```python
from build123d import *
from build123d.topology import SkipClean

# Parameters (mm, degrees)
SKETCH1_R           = 11.1
SKETCH1_R_2         = 2.95
BOSS_EXTRUDE1_DEPTH = 6.4
CUT_EXTRUDE4_REACH  = 48.556
CHAMFER1_SIZE       = 1
CUT_EXTRUDE3_DEPTH  = 47.555734529
FILLET1_R           = 10
FILLET2_R           = 5
SKETCH7_R           = 11.1
SKETCH7_R_2         = 9.1
BOSS_EXTRUDE2_DEPTH = 0.4
SKETCH9_OUTSIDE_W   = 87.68
SKETCH9_OUTSIDE_H   = 55.695
SKETCH9_OUTSIDE_R   = 16
CUT_EXTRUDE5_DEPTH  = 0.4
CUT_EXTRUDE6_DEPTH  = 0.15
CHAMFER2_SIZE       = 0.4


with BuildPart() as part:
    # Sketch1 → Boss-Extrude1 (new body)
    with BuildSketch(Plane(origin=(0, 0, 0), x_dir=(1, 0, 0), z_dir=(0, 1, 0))):
        with BuildLine():
            Line((-9.621787606, -11.507441213), (-37.944538575, 12.174234774))
            ThreePointArc((-37.944538575, 12.174234774), (-39.566706632, 19.240834224), (-33.200130557, 22.709979086))
            Line((-33.200130557, 22.709979086), (24.561921844, 13.989417946))
            ThreePointArc((24.561921844, 13.989417946), (29.443583706, 9.675962035), (27.514943911, 3.453673633))
            Line((27.514943911, 3.453673633), (9.621787606, -11.507441213))
            ThreePointArc((9.621787606, -11.507441213), (0, -15), (-9.621787606, -11.507441213))
        make_face()
        with Locations(Location((0, 0, 0), (0, 0, 270))):
            Circle(SKETCH1_R, mode=Mode.SUBTRACT)
        with Locations(Location((-34.095823533, 16.777211259, 0), (0, 0, 270))):
            Circle(SKETCH1_R_2, mode=Mode.SUBTRACT)
        with Locations(Location((23.666228869, 8.056650118, 0), (0, 0, 270))):
            Circle(SKETCH1_R_2, mode=Mode.SUBTRACT)
    extrude(amount=BOSS_EXTRUDE1_DEPTH)

    # Sketch6 → Cut-Extrude4 (cut, up to next)
    with BuildSketch(Plane(origin=(0, 6.4, 0), x_dir=(1, 0, 0), z_dir=(0, 1, 0)), mode=Mode.PRIVATE) as cut_extrude4_sk1:
        with BuildLine():
            Line((-10.397549699, 10.811612287), (-29.542980034, 22.157844884))
            Line((-29.542980034, 22.157844884), (21.066082003, 14.517198449))
            Line((21.066082003, 14.517198449), (11.313303216, 9.849323344))
            ThreePointArc((11.313303216, 9.849323344), (0.664192087, 14.985287747), (-10.397549699, 10.811612287))
        make_face()
    cut_extrude4_tool1 = extrude(cut_extrude4_sk1.sketch, amount=-CUT_EXTRUDE4_REACH, mode=Mode.PRIVATE) & part.part
    add(cut_extrude4_tool1.solids().sort_by_distance((-4.90649, 6.4, -15.955418))[0], mode=Mode.SUBTRACT)

    # Chamfer1
    chamfer1_edges = [part.edges().sort_by_distance(p)[0] for p in [
        (0, 6.4, -11.1),
    ]]
    chamfer(chamfer1_edges, length=CHAMFER1_SIZE)

    # Sketch5 → Cut-Extrude3 (cut, through all)
    with BuildSketch(Plane(origin=(0, 6.4, 0), x_dir=(1, 0, 0), z_dir=(0, 1, 0))):
        with BuildLine():
            Line((-37.944538575, 12.174234774), (-9.621787606, -11.507441213))
            ThreePointArc((-9.621787606, -11.507441213), (-21.736768022, 2.78083918), (-37.944538575, 12.174234774))
        make_face()
        with BuildLine():
            Line((9.621787606, -11.507441213), (27.514943911, 3.453673633))
            ThreePointArc((27.514943911, 3.453673633), (17.45368355, -2.69374898), (9.621787606, -11.507441213))
        make_face()
    extrude(amount=-CUT_EXTRUDE3_DEPTH, mode=Mode.SUBTRACT)

    # Fillet1
    fillet1_edges = [part.edges().sort_by_distance(p)[0] for p in [
        (-9.621787606, 3.2, 11.507441213),
        (9.621787606, 3.2, 11.507441213),
        (11.313303216, 3.2, -9.849323344),
        (-10.397549699, 3.2, -10.811612287),
        (-29.542980034, 3.2, -22.157844884),
        (21.066082003, 3.2, -14.517198449),
    ]]
    fillet(fillet1_edges, radius=FILLET1_R)

    # Fillet2
    fillet2_edges = [part.edges().sort_by_distance(p)[0] for p in [
        (-37.944538575, 3.2, -12.174234774),
        (27.514943911, 3.2, -3.453673633),
    ]]
    fillet(fillet2_edges, radius=FILLET2_R)

    # Sketch7 → Boss-Extrude2 (add)
    with BuildSketch(Plane.XZ):
        with Locations(Location((0, 0, 0), (0, 0, 270))):
            Circle(SKETCH7_R)
        with Locations(Location((0, 0, 0), (0, 0, 270))):
            Circle(SKETCH7_R_2, mode=Mode.SUBTRACT)
    extrude(amount=-BOSS_EXTRUDE2_DEPTH)

    # Sketch9 outside → Cut-Extrude5 (cut)
    with BuildSketch(Plane.XZ):
        with Locations((-5.215, -3.8885)):
            Rectangle(SKETCH9_OUTSIDE_W, SKETCH9_OUTSIDE_H)
        Circle(SKETCH9_OUTSIDE_R, mode=Mode.SUBTRACT)
    extrude(amount=-CUT_EXTRUDE5_DEPTH, mode=Mode.SUBTRACT)

    # Sketch10 → Cut-Extrude6 (cut)
    with SkipClean():  # the faces are left unmerged after this step: merging them gives an invalid solid
        with BuildSketch(Plane.XZ.offset(-0.4)):
            with BuildLine():
                Line((-33.200130557, -22.709979086), (-31.471010975, -22.448927195))
                ThreePointArc((-31.471010975, -22.448927195), (-29.606213483, -21.980449689), (-27.865545183, -21.16373999))
                Line((-27.865545183, -21.16373999), (-15.778990975, -14.000837254))
                ThreePointArc((-15.778990975, -14.000837254), (-12.899787471, -12.852921242), (-9.807384948, -12.641803688))
                ThreePointArc((-9.807384948, -12.641803688), (-14.988647226, -5.59825458), (-15.693394103, 3.11727149))
                ThreePointArc((-15.693394103, 3.11727149), (-25.389120558, -5.583543581), (-36.859243696, -11.759915461))
                ThreePointArc((-36.859243696, -11.759915461), (-38.564746422, -12.878937509), (-39.681392394, -14.585996871))
                ThreePointArc((-39.681392394, -14.585996871), (-38.786079998, -20.519068323), (-33.200130557, -22.709979086))
            make_face()
        extrude(amount=-CUT_EXTRUDE6_DEPTH, mode=Mode.SUBTRACT)

    # Chamfer2
    chamfer2_edges = [part.edges().sort_by_distance(p)[0] for p in [
        (9.181258422, 0, -12.186693797),
        (0.664192087, 0, -14.985287747),
        (-8.067073348, 0, -12.95119066),
        (12.787484872, 0, 7.295073573),
        (8.973593298, 0, 11.909370886),
        (0.284328537, 0, 14.997305001),
        (-8.853535866, 0, 11.952551059),
        (-13.030899461, 0, 6.394129067),
        (-8.853535866, 6.4, 11.952551059),
        (0.284328537, 6.4, 14.997305001),
        (-22.030616875, 6.4, -3.024808286),
        (8.973593298, 6.4, 11.909370886),
        (-38.564746422, 6.4, -12.878937509),
        (17.688730274, 6.4, 2.498737743),
        (-38.786079998, 6.4, -20.519068323),
        (28.054256045, 6.4, -4.038174832),
        (-32.335570766, 6.4, -22.579453141),
        (28.974894193, 6.4, -10.852731747),
        (-29.606213483, 6.4, -21.980449689),
        (24.33317404, 6.4, -14.023952889),
        (-21.822268079, 6.4, -17.582288622),
        (21.134254432, 6.4, -14.06081124),
        (-11.148337367, 6.4, -12.614536482),
        (17.625106381, 6.4, -12.870278654),
        (0.664192087, 6.4, -14.985287747),
        (12.220655249, 6.4, -11.578753904),
        (13.986327713, 0.4, -11.661249433),
        (17.625106381, 0.4, -12.870278654),
        (21.134254432, 0.4, -14.06081124),
        (20.643800798, 0.4, 0.286607853),
        (24.33317404, 0.4, -14.023952889),
        (28.054256045, 0.4, -4.038174832),
        (28.974894193, 0.4, -10.852731747),
        (-25.389120558, 0.55, -5.583543581),
        (-38.564746422, 0.55, -12.878937509),
        (-38.786079998, 0.55, -20.519068323),
        (-32.335570766, 0.55, -22.579453141),
        (-29.606213483, 0.55, -21.980449689),
        (-12.899787471, 0.55, -12.852921242),
        (-21.822268079, 0.55, -17.582288622),
    ]]
    chamfer(chamfer2_edges, length=CHAMFER2_SIZE)


with BuildPart() as body_2:
    # Mirror1: mirrored copy
    add(part.part.mirror(Plane.ZX))


solid = body_2.part
```
Geometry: final body of the model. Coordinates: model frame, mm. A direction names the side the tool comes from. Round coordinates to 2 decimals unless told otherwise and drop trailing zeros. Order: outer loops, then holes, each group sorted by start corner. A loop starts at its lowest first (then second) coordinate and runs counter-clockwise, first axis right, second up. Notation, with made-up numbers: (72, 13) -> (114, 13) arc R21 cw to (114, 31) -> close; hole circle Ø9 at (11, -37). An arc over 180 degrees is marked (long way). Use one line per item in the form item = value. Start each with the question number.
1. Line query: probe 1 along X at (y, z) = (-0.1, 0); probe 2 along Z at (x, y) = (-0.5, -3.5); probe 3 along X at (y, z) = (-5, -7.5). Output: solid intervals per line, ascending.
2. Pin query (flat end, axial travel): pin 1 Ø1 at (y, z) = (-4.5, -18) entering from +X; pin 2 Ø9 at (x, z) = (24.5, -1.5) entering from +Y; pin 3 Ø13.5 at (x, z) = (0, 0) entering from +Y; pin 4 Ø4 at (x, z) = (-19, -18) entering from -Y. Return the tip coordinate at first contact, or that it passes through.
3. Draft query along Z for faces 1 (the face through (-38.51, -6.29, -20.4)), 2 (the face through (17.634, -3.436, -12.875)), 3 (the face through (9.1, -0.4, 1.7)). Return one class per face: pulls with the +Z half, pulls with the -Z half, needs draft (parallel to the pull), parting line crosses it, or undercut.
4. Cut plane A-A (x = 0). Return the cut outline in (y, z), then the cut area to 3 significant figures.
5. Reachability of faces 4 (the face through (-22.01, -0.75, -17.46)), 5 (the face through (-29.714, -0.703, -21.756)) from +Z, -Z, +X, -X, +Y, -Y: full face, straight path, thin tool, end or side. Return the list, or none.
6. Cut plane B-B (y = -4). Count the separate pieces of the cut face and the enclosed holes in it, then the cut area to 3 significant figures.
Solution:
q1.probe_1 = -16 to -9.1, 9.1 to 16
q1.probe_2 = -14.99 to -11.09, 11.09 to 14.99
q1.probe_3 = -28.31 to -8.18, 8.18 to 20.77, 26.56 to 29.64
q2.pin_1 = -21.68
q2.pin_2 = -0.4
q2.pin_3 = through
q2.pin_4 = -6.2
q3.face_1 = parting line crosses it
q3.face_2 = pulls with the -Z half
q3.face_3 = undercut
q4.outline = (-6.4, -14.6) -> (-6, -15) -> (-0.4, -15) -> (0, -14.6) -> (0, -9.1) -> (-0.4, -9.1) -> (-0.4, -11.1) -> (-5.4, -11.1) -> (-6.4, -12.1) -> close; (-6.4, 12.1) -> (-5.4, 11.1) -> (-0.4, 11.1) -> (-0.4, 9.1) -> (0, 9.1) -> (0, 14.6) -> (-0.4, 15) -> (-6, 15) -> (-6.4, 14.6) -> close
q4.area = 50.2 mm^2
q5.face_4 = -Z, +Y
q5.face_5 = -Z, +X, +Y
q6.separate_pieces = 1
q6.enclosed_holes = 3
q6.area = 826 mm^2
